Model file for the job. Use its own axes, mm. A direction names the side the tool comes from. Coordinates: 2 decimals unless noted, no trailing zeros. Write each loop counter-clockwise with the first axis right and the second up, starting at its lowest first coordinate (ties: lowest second). Pieces come first, ordered by that corner, then holes.
Q1. Band-saw the part on B-B, the plane z = 38.1. Write the cut outline in (x, y) (3 decimals), plus the area to 3 significant figures.
Q2. Pull direction Z, two halves, no side cores. Call faces 6 (the flat face through (-18.2, 16, -1)), 7 (the flat face through (2, 2.5, -39)), 8 (the cylindrical face through (17.6, 16, -49.43)), 9 (the cylindrical face through (0.923, 6.302, -36.326)): released by +Z, released by -Z, zero draft, split by the parting line, or undercut.
Q3. Band-saw the part on A-A, the plane y = 22.5. Write the cut outline in (x, z).
Q4. Which spindle directions (+Z, -Z, +X, -X, +Y, -Y) get a long thin tool onto all of the face, cutting with end or side? Do faces 1 (the flat face through (16, 30.4, -1)), 2 (the flat face through (13.2, 18, -1)), 3 (the flat face through (18.2, 16, 1)), 4 (the cylindrical face through (-0.94, 6.73, 8.48)), 5 (the cylindrical face through (-0.65, 1.23, 35.17)). Say none if no direction does.
Q5. Drill centre lines: probe 1 along X at (y, z) = (6, 38.1) (3 decimals); probe 2 along X at (y, z) = (13, 15); probe 3 along Y at (x, z) = (3.5, -22). Where is each one in solid material? Low to high.
Q6. Band-saw the part on C-C, the plane x = 0. State how many separate pieces and enclosed holes the cut face has, plus the area to 3 significant figures.
Q7. Band-saw the part on D-D, the plane z = -1. Write the cut outline in (x, y).
Q8. Pin check, flat tips, straight feed: P1, Ø4, axis at x = 13, y = 15, coming from the -Z side; P2, Ø3.5, axis at x = 0, z = -38.1, coming from the +Y side; P3, Ø4.5, axis at x = 1.5, z = -13, coming from the +Y side; P4, Ø1.5, axis at x = -8.5, z = -11, coming from the +Y side. Stop position of each tip, or through.
Autodesk Inventor part; units mm, degrees
ref_plane "YZ Plane" through (0, 0, 0) normal (1, 0, 0) x (0, 1, 0)
ref_plane "XZ Plane" through (0, 0, 0) normal (0, 1, 0) x (-1, 0, 0)
ref_plane "XY Plane" through (0, 0, 0) normal (0, 0, 1) x (1, 0, 0)
sketch "Sketch1" plane through (0, 0, 0) normal (0, 1, 0) x (-1, 0, 0)
  line L0 (18.2, 50) -> (-18.2, 50)
  line L1 (-18.2, 50) -> (-18.2, -50)
  line L2 (-18.2, -50) -> (18.2, -50)
  line L3 (18.2, -50) -> (18.2, 50)
  point P0 (0, 0)
  dimension "d0" = 36.4
  dimension "d1" = 100
extrude "Extrusion1" add sketch "Sketch1" along normal blind 5
sketch "Sketch2" plane through (0, 5, 0) normal (0, 1, 0) x (1, 0, 0)
  circle A0 centre (0, 12.7) radius 4.325
  circle A1 centre (0, -12.7) radius 4.325
  circle A2 centre (0, -38.1) radius 4.325
  circle A3 centre (0, 38.1) radius 4.325
  point P0 (0, 0)
  dimension "d4" = 8.65
  dimension "d5" = 8.65
  dimension "d6" = 8.65
  dimension "d7" = 8.65
extrude "Extrusion2" add sketch "Sketch2" along normal blind 5
chamfer "Chamfer1" distance 1.5 angle 45 4 edges at (-4.325, 10, 38.1) (-4.325, 10, 12.7) (-4.325, 10, -12.7) (-4.325, 10, -38.1)
sketch "Sketch3" plane through (0, 5, 0) normal (0, 1, 0) x (1, 0, 0)
  line L0 (-18.2, 50) -> (-18.2, -50)
  line L1 (-18.2, -50) -> (18.2, -50)
  line L2 (-18.2, 50) -> (-13.2, 50)
  line L3 (-13.2, 50) -> (-13.2, -50)
  line L4 (-13.2, -50) -> (-18.2, -50)
  line L5 (-18.2, -50) -> (-18.2, 50)
  line L6 (18.2, -50) -> (18.2, 50)
  line L7 (18.2, 50) -> (13.2, 50)
  line L8 (13.2, 50) -> (13.2, -50)
  line L9 (13.2, -50) -> (18.2, -50)
  line L10 (18.2, -50) -> (18.2, 50)
  point P0 (0, 0)
  dimension "d13" = 5
  dimension "d14" = 5
extrude "Extrusion3" add sketch "Sketch3" along normal blind 25.4
sketch "Sketch4" plane through (0, 10, 38.1) normal (0, 1, 0) x (1, 0, 0)
  circle A0 centre (0, 0) radius 2.825
  circle A1 centre (0, 0) radius 2
  circle A2 centre (0, 25.4) radius 2.825
  circle A3 centre (0, 25.4) radius 2
  circle A4 centre (0, 50.8) radius 2.825
  circle A5 centre (0, 50.8) radius 2
  circle A6 centre (0, 76.2) radius 2.825
  circle A7 centre (0, 76.2) radius 2
  point P0 (0, 38.1)
  dimension "d17" = 4
  dimension "d18" = 4
  dimension "d19" = 4
  dimension "d20" = 4
extrude "Extrusion4" cut sketch "Sketch4" against normal blind 25.4 contours A1 | A3 | A5 | A7
sketch "Sketch5" plane through (0, 0, 0) normal (0, -1, 0) x (1, 0, 0)
  circle A0 centre (0, 38.1) radius 2.825
  circle A1 centre (0, 38.1) radius 3
  circle A2 centre (0, 12.7) radius 2
  circle A3 centre (0, 12.7) radius 3
  circle A4 centre (0, -12.7) radius 3
  circle A5 centre (0, -38.1) radius 2
  circle A6 centre (0, -38.1) radius 3
  point P0 (0, 0)
  dimension "d23" = 6
  dimension "d24" = 6
  dimension "d25" = 6
  dimension "d26" = 6
extrude "Extrusion5" cut sketch "Sketch5" against normal blind 2.5 contours A0 | A1 | A2 | A3 | A4 | A5 | A6
fillet "Fillet1" radius 2 8 edges at (-18.2, 0, 0) (0, 0, 50) (18.2, 0, 0) (0, 0, -50) (-18.2, 15.2, -50) (-18.2, 15.2, 50) (18.2, 15.2, 50) (18.2, 15.2, -50)
properties part number "CBCaseMount"
Answer sheet:
1. outline: (-18.2, 2) arc R2 ccw to (-16.2, 0) - (-3, 0) - (-3, 2.5) - (-2, 2.5) - (-2, 10) - (-2.825, 10) - (-4.325, 8.5) - (-4.325, 5) - (-13.2, 5) - (-13.2, 30.4) - (-18.2, 30.4) - close; (2, 2.5) - (3, 2.5) - (3, 0) - (16.2, 0) arc R2 ccw to (18.2, 2) - (18.2, 30.4) - (13.2, 30.4) - (13.2, 5) - (4.325, 5) - (4.325, 8.5) - (2.825, 10) - (2, 10) - close
1. area: 430 mm2
2. face 6: zero draft
2. face 7: undercut
2. face 8: released by -Z
2. face 9: undercut
3. outline: (-18.2, -48) arc R2 ccw to (-16.2, -50) - (-13.2, -50) - (-13.2, 50) - (-16.2, 50) arc R2 ccw to (-18.2, 48) - close; (13.2, -50) - (16.2, -50) arc R2 ccw to (18.2, -48) - (18.2, 48) arc R2 ccw to (16.2, 50) - (13.2, 50) - close
4. face 1: +Z, -Z, +X, -X, +Y
4. face 2: +Z, -Z, +Y
4. face 3: +Z, -Z, +X, +Y, -Y
4. face 4: +Y
4. face 5: -Y
5. probe 1: x = -18.2 to -13.2, -4.325 to -2, 2 to 4.325, 13.2 to 18.2
5. probe 2: x = -18.2 to -13.2, 13.2 to 18.2
5. probe 3: y = 0 to 5
6. separate pieces: 5
6. enclosed holes: 0
6. area: 482 mm2
7. outline: (-18.2, 2) arc R2 ccw to (-16.2, 0) - (16.2, 0) arc R2 ccw to (18.2, 2) - (18.2, 30.4) - (13.2, 30.4) - (13.2, 5) - (-13.2, 5) - (-13.2, 30.4) - (-18.2, 30.4) - close
8. P1: stops at z = -50
8. P2: passes through
8. P3: stops at y = 10
8. P4: stops at y = 5
